Here's how the part is built. I have some questions about the finished solid (model axes, mm). Coordinates: 2 decimals unless noted, no trailing zeros. Loops run counter-clockwise (first coordinate to the right, second up) from the corner with the lowest first, then second, coordinate; pieces in that order, holes last. Notation, with made-up numbers: (50.5, 48) -> (57.5, 48) arc R21 ccw to (57.5, 62) -> close; hole circle Ø8 at (-31.75, 51.25). An arc over 180 degrees is marked (long way). Answer as a JSON object with one key per item and string values. Group by question number.
1) I want a section at B-B (y = 0). Write out the boundary of the cut face in (x, z), then the cut area to 3 significant figures.
2) I'm going to push flat-ended pins straight in: pin 1 (1.5 mm diameter, centred on x = 11, z = 0.5, fed in from +Y); pin 2 (0.9 mm diameter, centred on x = 0.5, z = 1.5, fed in from +Y); pin 3 (4 mm diameter, centred on x = 0, y = 62, fed in from -Z); pin 4 (1 mm diameter, centred on x = 46.5, z = 0.5, fed in from +Y). Where does each tip first touch, or does it pass through?
3) I need wall thicknesses on probe 1 along X at (y, z) = (23, 1.3); probe 2 along X at (y, z) = (-21.5, 0.7) (3 decimals); probe 3 along X at (y, z) = (-15, 0.8). Which ranges of each line are inside material? Lowest first, please. Write a range as [from, to].
4) If we mould it in two halves opening along X, with no side actions, what happens to faces 1 (the cylindrical face through (-9.373, 71.387, 1.479)), 2 (the flat face through (-1, 17, 0)), 3 (the cylindrical face through (64.056, -9.767, 1.521))? For each: +X half, -X half, draft (parallel to the pull), parting line (faces both ways), or undercut.
5) I want a section at D-D (y = 62). Write out the boundary of the cut face in (x, z).
6) I want a section at C-C (x = -54). Write out the boundary of the cut face in (y, z).
7) I want a section at A-A (z = 2). Write out the boundary of the cut face in (x, y).
```python
from build123d import *

# Parameters (mm, degrees)
F0_R     = 72
F1_DEPTH = 3
F2_R     = 25.5
F3_DEPTH = 3
F4_R     = 2.5
F5_DEPTH = 25.4
F6_W     = 20
F6_H     = 41
F7_DEPTH = 3
F8_R     = 2.5
F9_DEPTH = 25.4


with BuildPart() as f1:
    # F0 (on Top) → F1 (new body)
    with BuildSketch(Plane.XY):
        Circle(F0_R)
    extrude(amount=F1_DEPTH)

    # F2 (on face) → F3 (cut)
    with BuildSketch(Plane.XY.offset(3)):
        with Locations((-40.5, 0)):
            Circle(F2_R)
        with Locations((40.5, 0)):
            Circle(F2_R)
    extrude(amount=-F3_DEPTH, mode=Mode.SUBTRACT)

    # F4 (on face) → F5 (cut)
    with BuildSketch(Plane.XY.offset(3)):
        with Locations((0, 62)):
            Circle(F4_R)
        Circle(F4_R)
        with Locations((0, -64)):
            Circle(F4_R)
    extrude(amount=-F5_DEPTH, mode=Mode.SUBTRACT)

    # F6 (on face) → F7 (cut)
    with BuildSketch(Plane.XY.offset(3)):
        with Locations((0, -10.5)):
            Rectangle(F6_W, F6_H)
    extrude(amount=-F7_DEPTH, mode=Mode.SUBTRACT)

    # F8 (on face) → F9 (cut)
    with BuildSketch(Plane.XY.offset(3)):
        with Locations((-53.693575, -31)):
            Circle(F8_R)
        with Locations((53.693575, -31)):
            Circle(F8_R)
    extrude(amount=-F9_DEPTH, mode=Mode.SUBTRACT)


solid = f1.part
```
Determined:
{
 "1": {"outline": "(-72, 0) -> (-66, 0) -> (-66, 3) -> (-72, 3) -> close; (-15, 0) -> (-10, 0) -> (-10, 3) -> (-15, 3) -> close; (10, 0) -> (15, 0) -> (15, 3) -> (10, 3) -> close; (66, 0) -> (72, 0) -> (72, 3) -> (66, 3) -> close", "area": "66.0 mm^2"},
 "2": {"pin 1": "y = 71.27", "pin 2": "y = 72", "pin 3": "through", "pin 4": "y = 55.39"},
 "3": {"probe 1": "[-68.23, -51.51], [-29.49, 29.49], [51.51, 68.23]", "probe 2": "[-68.715, -54.211], [-26.789, -10], [10, 26.789], [54.211, 68.715]", "probe 3": "[-70.42, -61.12], [-19.88, -10], [10, 19.88], [61.12, 70.42]"},
 "4": {"face 1": "parting line", "face 2": "draft", "face 3": "undercut"},
 "5": {"outline": "(-36.61, 0) -> (-2.5, 0) -> (-2.5, 3) -> (-36.61, 3) -> close; (2.5, 0) -> (36.61, 0) -> (36.61, 3) -> (2.5, 3) -> close"},
 "6": {"outline": "(-47.62, 0) -> (-33.48, 0) -> (-33.48, 3) -> (-47.62, 3) -> close; (-28.52, 0) -> (-21.63, 0) -> (-21.63, 3) -> (-28.52, 3) -> close; (21.63, 0) -> (47.62, 0) -> (47.62, 3) -> (21.63, 3) -> close"},
 "7": {"outline": "circle Ø144 at (0, 0); hole circle Ø51 at (-40.5, 0); hole circle Ø5 at (-53.69, -31); hole (-10, -31) -> (10, -31) -> (10, 10) -> (-10, 10) -> close; hole circle Ø5 at (0, -64); hole circle Ø5 at (0, 62); hole circle Ø51 at (40.5, 0); hole circle Ø5 at (53.69, -31)"}
}
